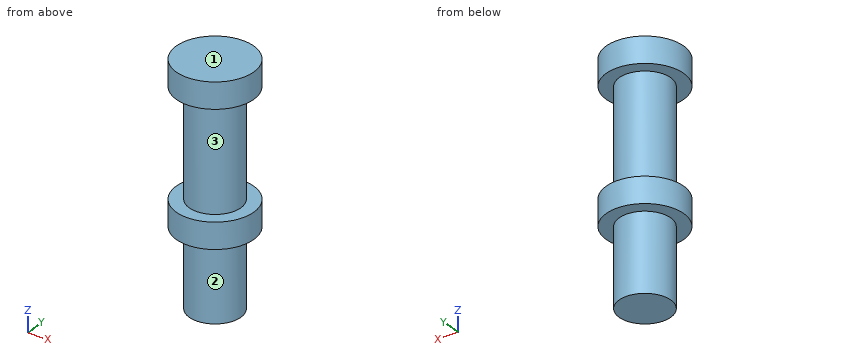
from build123d import *

# Parameters (mm, degrees)
SKETCH1_R               = 1
BOSS_EXTRUDE1_DEPTH     = 9.12
BOSS_EXTRUDE2_START     = 3
BOSS_EXTRUDE2_OUTLINE_R = 1.5
BOSS_EXTRUDE2_DEPTH     = 1
BOSS_EXTRUDE3_START     = -1
SKETCH2_R               = 1.5
BOSS_EXTRUDE3_DEPTH     = 1


# Read off the part's stored shape, not the designer's step: Boss-Extrude2
with BuildPart() as part:
    # Sketch1 → Boss-Extrude1 (new body)
    with BuildSketch(Plane.XY):
        Circle(SKETCH1_R)
    extrude(amount=BOSS_EXTRUDE1_DEPTH)

    # Boss-Extrude2 outline → Boss-Extrude2 (add)
    with BuildSketch(Plane.XY.offset(BOSS_EXTRUDE2_START)):
        Circle(BOSS_EXTRUDE2_OUTLINE_R)
    extrude(amount=BOSS_EXTRUDE2_DEPTH)

    # Sketch2 → Boss-Extrude3 (add)
    with BuildSketch(Plane.XY.offset(9.12).offset(BOSS_EXTRUDE3_START)):
        Circle(SKETCH2_R)
    extrude(amount=BOSS_EXTRUDE3_DEPTH)


solid = part.part
Source: CAD feature listing. Evaluate the final solid. Frame: model axes, mm. Face numbers are marked on the shaded views. A direction names the side the tool comes from. Give positions to 0.01 mm unless a question says otherwise; leave off trailing zeros. Write each loop counter-clockwise with the first axis right and the second up, starting at its lowest first coordinate (ties: lowest second). Pieces come first, ordered by that corner, then holes. Notation, with made-up numbers: M 5,12.5 L 22,12.5 A31 cw 22,37.5 Z; hole C 12,41.5 d9. An arc over 180 degrees is marked long. Return JSON: item names as keys, results as strings. Group by question number.
1) Set-up query: the marked faces 1, 2 and 3. Return all of +Z, -Z, +X, -X, +Y, -Y with unobstructed straight access to the full face (end or side cutting, diameter ignored); none if empty.
2) Ray query, L1, parallel to Z at x = -0.45, y = 1.35; L2, parallel to X at y = -0.05, z = 1.75; L3, parallel to Y at x = 0.1, z = 4.5. Return the intervals inside material, ascending.
3) Cut plane A-A, the plane x = -1.2. Output: boundary loops of the cut face in (y, z), then the cut area to 3 significant figures.
4) Cut plane D-D, the plane z = 3.5. Output: boundary loops of the cut face in (x, y), then the cut area to 3 significant figures.
5) First-contact query: pin 1 Ø1.5 at (y, z) = (0.5, 5.5) entering from -X. Flat tip, straight axial feed; report the tip coordinate or a pass-through.
6) Cut plane B-B, the plane y = 1.25. Output: boundary loops of the cut face in (x, z).
7) Cut plane C-C, the plane y = 0. Output: boundary loops of the cut face in (x, z), then the cut area to 3 significant figures.
Data:
{
 "1": {"face 1": "+Z, +X, -X, +Y, -Y", "face 2": "-Z", "face 3": "none"},
 "2": {"L1": "z = 3 to 4, 8.12 to 9.12", "L2": "x = -1 to 1", "L3": "y = -0.99 to 0.99"},
 "3": {"outline": "M -0.9,3 L 0.9,3 L 0.9,4 L -0.9,4 Z; M -0.9,8.12 L 0.9,8.12 L 0.9,9.12 L -0.9,9.12 Z", "area": "3.60 mm²"},
 "4": {"outline": "C 0,0 d3", "area": "7.07 mm²"},
 "5": {"pin 1": "stops at x = -1"},
 "6": {"outline": "M -0.83,3 L 0.83,3 L 0.83,4 L -0.83,4 Z; M -0.83,8.12 L 0.83,8.12 L 0.83,9.12 L -0.83,9.12 Z"},
 "7": {"outline": "M -1.5,3 L -1,3 L -1,0 L 1,0 L 1,3 L 1.5,3 L 1.5,4 L 1,4 L 1,8.12 L 1.5,8.12 L 1.5,9.12 L -1.5,9.12 L -1.5,8.12 L -1,8.12 L -1,4 L -1.5,4 Z", "area": "20.2 mm²"}
}
